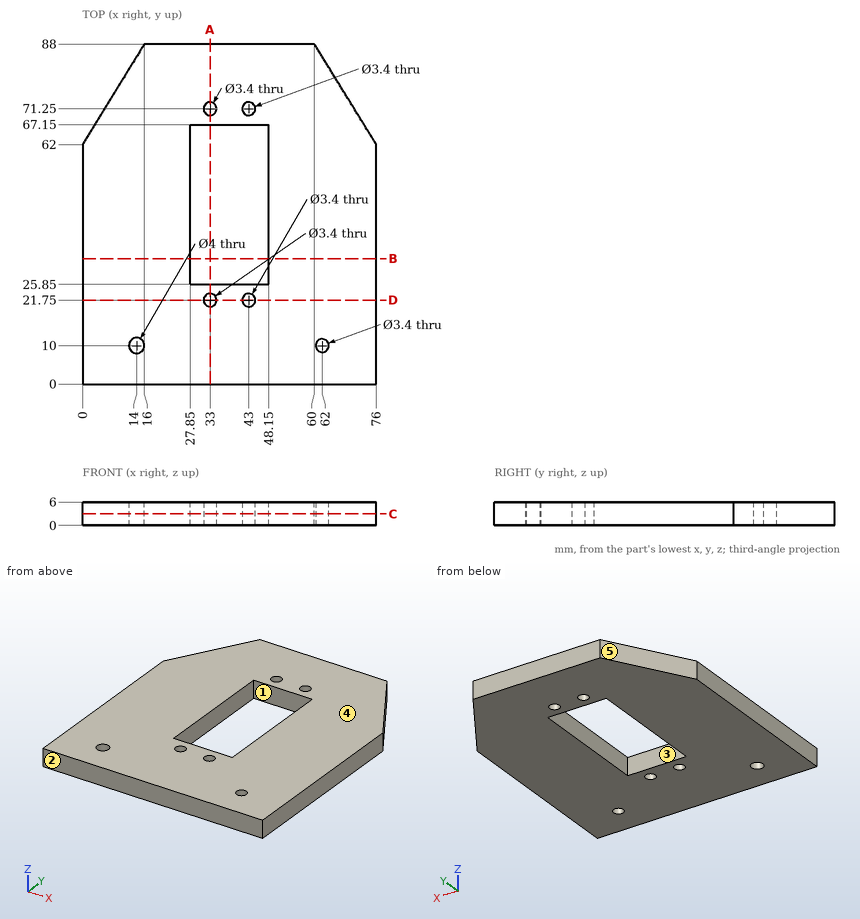
Drawing for the job (mm, zero at the part's lowest x, y, z). A direction names the side the tool comes from. Give positions to 0.01 mm unless a question says otherwise; leave off trailing zeros. Order: outer loops, then holes, each group sorted by start corner. A loop starts at its lowest first (then second) coordinate and runs counter-clockwise, first axis right, second up. Notation, with made-up numbers: M 31.25,-23.5 L 67.25,-23.5 A8 cw 67.25,-8.5 Z; hole C -33.75,80 d2. An arc over 180 degrees is marked long. Write item = value, one per line. Start each with the question number.
(1) Slice it at A-A on x = 33. Write the cut outline in (y, z).
(2) Slice it at C-C on z = 2.95. Write the cut outline in (x, y), plus the area to 3 significant figures.
(3) Probe L1, parallel to Y at x = 38.5, z = 1.4; L2, parallel to X at y = 70, z = 3.45; L3, parallel to X at y = 47, z = 4.2. List the from-to ranges inside material, lowest first. Write a range as [from, to].
(4) Two-plate mould, pull along X, no slides. Class the marked faces 3, 4 and 5: released by +X, released by -X, zero draft, split by the parting line, or undercut.
(5) Which spindle directions (+Z, -Z, +X, -X, +Y, -Y) get a long thin tool onto all of the face, cutting with end or side? Do the marked faces 1 and 2. Say none if no direction does.
(6) Slice it at B-B on y = 32.5. Write the cut outline in (x, z).
(7) Slice it at D-D on y = 21.75. Write the cut outline in (x, z), plus the area to 3 significant figures.
Responses:
q1.outline = M 0,0 L 20.05,0 L 20.05,6 L 0,6 Z; M 23.45,0 L 25.85,0 L 25.85,6 L 23.45,6 Z; M 67.15,0 L 69.55,0 L 69.55,6 L 67.15,6 Z; M 72.95,0 L 88,0 L 88,6 L 72.95,6 Z
q2.outline = M 0,0 L 76,0 L 76,62 L 60,88 L 16,88 L 0,62 Z; hole C 14,10 d4; hole M 27.85,25.85 L 48.15,25.85 L 48.15,67.15 L 27.85,67.15 Z; hole C 33,21.75 d3.4; hole C 33,71.25 d3.4; hole C 43,21.75 d3.4; hole C 43,71.25 d3.4; hole C 62,10 d3.4
q2.area = 5,380 mm2
q3.L1 = [0, 25.85], [67.15, 88]
q3.L2 = [4.92, 31.85], [34.15, 41.85], [44.15, 71.08]
q3.L3 = [0, 27.85], [48.15, 76]
q4.face_3 = undercut
q4.face_4 = zero draft
q4.face_5 = released by -X
q5.face_1 = +Z, -Z
q5.face_2 = +Z, -Z, +X, -X, -Y
q6.outline = M 0,0 L 27.85,0 L 27.85,6 L 0,6 Z; M 48.15,0 L 76,0 L 76,6 L 48.15,6 Z
q7.outline = M 0,0 L 31.3,0 L 31.3,6 L 0,6 Z; M 34.7,0 L 41.3,0 L 41.3,6 L 34.7,6 Z; M 44.7,0 L 76,0 L 76,6 L 44.7,6 Z
q7.area = 415 mm2
